Verification items for the finished model (mm, model axes). A direction names the side the tool comes from. Coordinates: 2 decimals unless noted, no trailing zeros. Order: outer loops, then holes, each group sorted by start corner. A loop starts at its lowest first (then second) coordinate and runs counter-clockwise, first axis right, second up. Notation, with made-up numbers: (29.25, 29.25) - (74.25, 29.25) arc R12 cw to (74.25, 46.25) - close; hole circle Ø5 at (-37, -21). An arc over 180 degrees is marked (long way). Answer as CSV lines item,"result". Start each with the question number.
1. Go/stop test with flat-tipped pins: pin 1 (8 mm diameter, centred on x = 19.5, y = 5.5, fed in from -Z); pin 2 (2 mm diameter, centred on y = -6, z = 1.5, fed in from +X); pin 3 (1 mm diameter, centred on x = 13.5, y = -3.5, fed in from +Z); pin 4 (2 mm diameter, centred on x = 9, z = 6.5, fed in from -Y). Record where each tip stops, or that it passes through.
2. Set-up check for faces 1 (the cylindrical face through (27.848, 3.233, -1.341)), 2 (the cylindrical face through (27, -3, 0)), 3 (the cylindrical face through (-3.169, -0.867, 3.905)): record each of +Z, -Z, +X, -X, +Y, -Y from which the full face is reachable in a straight line by a thin tool's end or side.
3. Mould release check, pull along X, two halves, no side actions. Record for faces 4 (the cylindrical face through (18.612, 3.233, -1.341)), 5 (the flat face through (3.5, 4, 4)), 6 (the flat face through (26.5, 3, -1)): pulls with the +X half, pulls with the -X half, needs draft (parallel to the pull), parting line crosses it, or undercut.
4. Material ranges on L1, parallel to X at y = 4.25, z = -3.5; L2, parallel to X at y = 4, z = -1.5; L3, parallel to Y at x = 26, z = 2.25, recorded low to high. Write a range as [from, to].
5. Section check C-C (x = 13). Record the cut outline in (y, z), and give its area (3 significant figures).
Autodesk Inventor part; units mm, degrees
ref_plane "YZ Plane" through (0, 0, 0) normal (1, 0, 0) x (0, 1, 0)
ref_plane "XZ Plane" through (0, 0, 0) normal (0, 1, 0) x (-1, 0, 0)
ref_plane "XY Plane" through (0, 0, 0) normal (0, 0, 1) x (1, 0, 0)
sketch "Skizze1" plane through (0, 0, 0) normal (0, 0, 1) x (1, 0, 0)
  line L0 (0, 0) -> (0, 10)
  line L1 (0, 10) -> (3.5, 10)
  line L2 (3.5, 10) -> (3.5, 5)
  line L3 (10.5, 3.5) -> (26.5, 3.5)
  line L4 (26.5, 3.5) -> (26.5, 3)
  line L5 (26.5, 3) -> (27.24, 3)
  line L6 (27.24, 3) -> (27.24, 3.5)
  line L7 (27.24, 3.5) -> (28.44, 3.5)
  line L8 (28.64, 3.3) -> (28.64, 0)
  line L9 (28.64, 0) -> (0, 0)
  line L10 (28.44, 3.5) -> (28.64, 3.3)
  line L11 (3.5, 5) -> (10.5, 5)
  line L12 (10.5, 5) -> (10.5, 3.5)
  line L13 (0, 4) -> (-7.5, 4)
  line L14 (-7.5, 4) -> (-7.5, 0)
  line L15 (-7.5, 0) -> (0, 0)
  point P0 (28.64, 3.5)
  dimension "d0" = 6
  dimension "d1" = 7
  dimension "d2" = 0.74
  dimension "d3" = 0.2
  dimension "d4" = 0.2
  dimension "d5" = 1.2
  dimension "d6" = 10
  dimension "d7" = 23
  dimension "d8" = 16
  dimension "d9" = 20
  dimension "Gabel_FixationShaft_Contact_Thickness" = 3.5
  dimension "d29" = 8
  dimension "d30" = 7.5
revolve "Umdrehung1" add sketch "Skizze1" angle 360 about axis through (28.64, 0, 0) along (-1, 0, 0)
chamfer "Fase1" distance 0.2 angle 45 3 edges at (10.5, -5, 0) (3.5, -10, 0) (0, -10, 0)
chamfer "Fase2" distance 1.25 angle 45 1 edges at (-7.5, -4, 0)
thread "Gewinde1"
properties part number "ParallelMecha_Gabel_Connection_JointShaft_Nadellager" material "Edelstahl"
Evaluation:
1,pin 1,"stops at z = -3.16"
1,pin 2,"stops at x = 3.5"
1,pin 3,"stops at z = 1.8"
1,pin 4,"passes through"
2,face 1,"+X"
2,face 2,"none"
2,face 3,"-X"
3,face 4,"needs draft"
3,face 5,"pulls with the +X half"
3,face 6,"undercut"
4,L1,"x = [0, 3.5]"
4,L2,"x = [0, 10.5]"
4,L3,"y = [-2.68, 2.68]"
5,outline,"circle Ø7 at (0, 0)"
5,area,"38.5 mm²"
